Here's how the part is built. I have some questions about the finished solid (model axes, mm). A direction names the side the tool comes from. Round coordinates to 2 decimals unless told otherwise and drop trailing zeros. Loops run counter-clockwise (first coordinate to the right, second up) from the corner with the lowest first, then second, coordinate; pieces in that order, holes last. Notation, with made-up numbers: M 33,18 L 45,18 A21 ccw 45,48 Z; hole C 17,42 d7. An arc over 180 degrees is marked long. Use a Markdown table: item, result.
from build123d import *

# Parameters (mm, degrees)
F0_W       = 10
F0_H       = 10
F0_W_2     = 5
F0_H_2     = 5
F1_DEPTH   = 50
F2_W       = 5
F2_H       = 5
F1_FACE1_W = 10
F1_FACE1_H = 50
F3_DEPTH   = 3
F4_W       = 5
F4_H       = 5
F5_DEPTH   = 4


with BuildPart() as f1:
    # F0 (on Top) → F1 (new body)
    with BuildSketch(Plane.XY):
        Rectangle(F0_W, F0_H)
        Rectangle(F0_W_2, F0_H_2, mode=Mode.SUBTRACT)
    extrude(amount=F1_DEPTH)

    # F2 (on face) + F1_face1 (on face) → F3 (cut)
    with BuildSketch(Plane.YZ.offset(5)):
        with Locations((0, 5.5)):
            Rectangle(F2_W, F2_H)
    with BuildSketch(Plane(origin=(-5, 0, 25), x_dir=(0, -1, 0), z_dir=(-1, 0, 0))):
        Rectangle(F1_FACE1_W, F1_FACE1_H)
    extrude(amount=-F3_DEPTH, dir=(1, 0, 0), mode=Mode.SUBTRACT)

    # F4 (on face) → F5 (cut)
    with BuildSketch(Plane(origin=(-5, 0, 0), x_dir=(0, -1, 0), z_dir=(-1, 0, 0))):
        with Locations((0, 42.5)):
            Rectangle(F4_W, F4_H)
    extrude(amount=-F5_DEPTH, mode=Mode.SUBTRACT)


solid = f1.part
1. Imagine slicing it at B-B, the plane y = -1.75. Write out the boundary of the cut face in (x, z).
Answer sheet:
| item | result |
|---|---|
| outline | M -5,0 L -2.5,0 L -2.5,40 L -5,40 Z; M -5,45 L -2.5,45 L -2.5,50 L -5,50 Z; M 2.5,0 L 5,0 L 5,3 L 2.5,3 Z; M 2.5,8 L 5,8 L 5,50 L 2.5,50 Z |
2. We'd pull the mould along Y, two halves only. Please class faces 1 (the face through (-4, 0, 40)), 2 (the face through (-2.5, 0, 20)), 3 (the face through (-5, 0, 25)), 4 (the face through (0, -5, 25)): +Y half, -Y half, draft (parallel to the pull), parting line (faces both ways), or undercut.
Answer sheet:
| item | result |
|---|---|
| face 1 | undercut |
| face 2 | undercut |
| face 3 | draft |
| face 4 | -Y half |
3. Imagine slicing it at A-A, the plane x = -0.25. Write out the boundary of the cut face in (y, z).
Answer sheet:
| item | result |
|---|---|
| outline | M -5,0 L -2.5,0 L -2.5,50 L -5,50 Z; M 2.5,0 L 5,0 L 5,50 L 2.5,50 Z |
4. I need wall thicknesses on probe 1 along Y at (x, z) = (0, 42); probe 2 along Z at (x, y) = (-4.5, 2); probe 3 along Z at (x, y) = (2.75, -2). Which ranges of each line are inside material? Lowest first, please. Write a range as from..to.
Answer sheet:
| item | result |
|---|---|
| probe 1 | -5..-2.5, 2.5..5 |
| probe 2 | 0..40, 45..50 |
| probe 3 | 0..3, 8..50 |
5. Which directions (+Z, -Z, +X, -X, +Y, -Y) give clear straight access to the entire face, cutting with the end or side of a thin tool? Please do faces 5 (the face through (-4, 0, 45)), 6 (the face through (-2.5, 0, 47)), 7 (the face through (4, 0, 8)).
Answer sheet:
| item | result |
|---|---|
| face 5 | -X |
| face 6 | +Z, -Z |
| face 7 | +X |
6. Imagine slicing it at C-C, the plane z = 31. Write out the boundary of the cut face in (x, y).
Answer sheet:
| item | result |
|---|---|
| outline | M -5,-5 L 5,-5 L 5,5 L -5,5 Z; hole M -2.5,-2.5 L 2.5,-2.5 L 2.5,2.5 L -2.5,2.5 Z |
7. Imagine slicing it at D-D, the plane x = -3.25. Write out the boundary of the cut face in (y, z).
Answer sheet:
| item | result |
|---|---|
| outline | M -5,0 L 5,0 L 5,50 L -5,50 Z; hole M -2.5,40 L 2.5,40 L 2.5,45 L -2.5,45 Z |
